Model file for the job. Use its own axes, mm. Face numbers are marked on the shaded views. Coordinates: 2 decimals unless noted, no trailing zeros. Loops run counter-clockwise (first coordinate to the right, second up) from the corner with the lowest first, then second, coordinate; pieces in that order, holes last. Notation, with made-up numbers: (45.25, 72.25) -> (94.25, 72.25) arc R10 ccw to (94.25, 89.25) -> close; hole circle Ø5 at (84, 87). An arc over 180 degrees is marked (long way). Use one line per item in the form item = value.
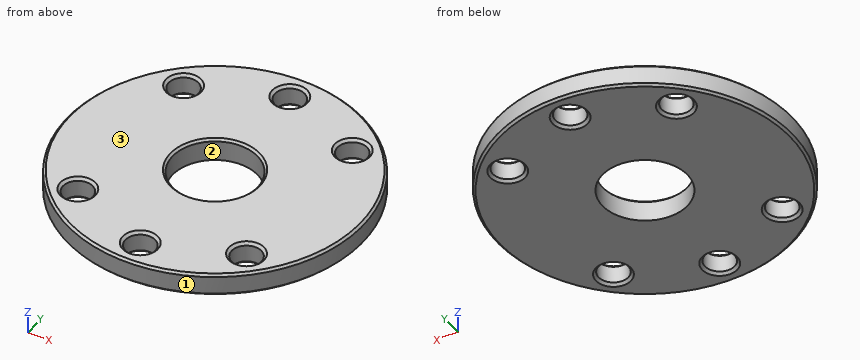
Solid Edge part; units mm, degrees
sketch "Sketch1" plane through (0, 0, 102) normal (0, 0, 1) x (1, 0, 0)
  circle A0 centre (0, 0) radius 33
  circle A1 centre (0, 0) radius 9.5
extrude "Protrusion1" add sketch "Sketch1" along normal blind 5
chamfer "Faza_1" distance 0.5 angle 45 3 edges at (-9.5, 0, 107) (-33, 0, 107) (-33, 0, 102)
hole "Otwór_1" at (-19.0919, 19.0919, 107) direction (0, 0, -1) diameter 6.647 end up to next start chamfer 0.6 start chamfer angle 45 end chamfer 0.6 end chamfer angle 45
hole "Hole1" at (0, 27, 107) direction (0, 0, -1) diameter 6.647 end up to next start chamfer 0.6 start chamfer angle 45 end chamfer 0.6 end chamfer angle 45
hole "Hole2" at (19.0919, 19.0919, 107) direction (0, 0, -1) diameter 6.647 end up to next start chamfer 0.6 start chamfer angle 45 end chamfer 0.6 end chamfer angle 45
hole "Hole3" at (19.0919, -19.0919, 107) direction (0, 0, -1) diameter 6.647 end up to next start chamfer 0.6 start chamfer angle 45 end chamfer 0.6 end chamfer angle 45
hole "Hole4" at (0, -27, 107) direction (0, 0, -1) diameter 6.647 end up to next start chamfer 0.6 start chamfer angle 45 end chamfer 0.6 end chamfer angle 45
hole "Hole5" at (-19.0919, -19.0919, 107) direction (0, 0, -1) diameter 6.647 end up to next start chamfer 0.6 start chamfer angle 45 end chamfer 0.6 end chamfer angle 45
Q1. Band-saw the part on B-B, the plane y = 0. Write the cut outline in (x, z), and give its area (3 significant figures).
Result:
outline = (-33, 102.5) -> (-32.5, 102) -> (-9.5, 102) -> (-9.5, 106.5) -> (-10, 107) -> (-32.5, 107) -> (-33, 106.5) -> close; (9.5, 102) -> (32.5, 102) -> (33, 102.5) -> (33, 106.5) -> (32.5, 107) -> (10, 107) -> (9.5, 106.5) -> close
area = 234 mm2
Q2. Pin check, flat tips, straight feed: pin 1 Ø4 at (x, y) = (19.09, -19.09) entering from +Z; pin 2 Ø1 at (y, z) = (12, 105) entering from -X; pin 3 Ø1.5 at (y, z) = (24, 106.5) entering from +X; pin 4 Ø7.5 at (x, y) = (-19.09, -19.09) entering from +Z. Stop position of each tip, or through.
Result:
pin_1 = through
pin_2 = -30.93
pin_3 = 23.42
pin_4 = 106.83
Q3. Mould opens along X. For the marked faces 1, 2 and 3 say: released by +X, released by -X, zero draft, split by the parting line, or undercut.
Result:
face_1 = split by the parting line
face_2 = undercut
face_3 = zero draft
Q4. Band-saw the part on C-C, the plane z = 104.75. Write the cut outline in (x, y), and give its area (3 significant figures).
Result:
outline = circle Ø66 at (0, 0); hole circle Ø6.65 at (-19.09, -19.09); hole circle Ø6.65 at (-19.09, 19.09); hole circle Ø19 at (0, 0); hole circle Ø6.65 at (0, -27); hole circle Ø6.65 at (0, 27); hole circle Ø6.65 at (19.09, -19.09); hole circle Ø6.65 at (19.09, 19.09)
area = 2,930 mm2
Q5. Wall check: line 1 along Y through (x, z) = (-1.5, 105.3); line 2 along X through (y, z) = (-27, 105.5); line 3 along X through (y, z) = (5, 102.6). Give the ranges that are in metal, low to high.
Result:
line_1 = -32.97 to -29.97, -24.03 to -9.38, 9.38 to 24.03, 29.97 to 32.97
line_2 = -18.97 to -3.32, 3.32 to 18.97
line_3 = -32.62 to -8.08, 8.08 to 32.62
Q6. Band-saw the part on A-A, the plane x = 0. State how many separate pieces and enclosed holes the cut face has, and give its area (3 significant figures).
Result:
separate_pieces = 4
enclosed_holes = 0
area = 166 mm2
